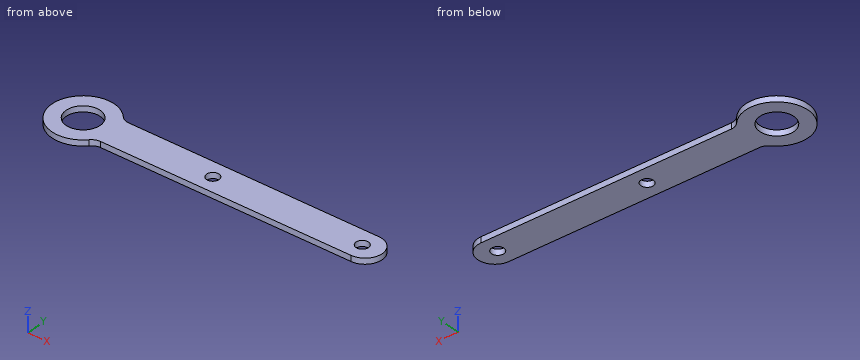
Autodesk Inventor part; units mm, degrees
ref_plane "YZ Plane" through (0, 0, 0) normal (1, 0, 0) x (0, 1, 0)
ref_plane "XZ Plane" through (0, 0, 0) normal (0, 1, 0) x (-1, 0, 0)
ref_plane "XY Plane" through (0, 0, 0) normal (0, 0, 1) x (1, 0, 0)
sketch "Skizze1" plane through (0, 0, 0) normal (0, 0, 1) x (1, 0, 0)
  line L0 (0, 0) -> (38.7995, 0) construction
  arc A0 (4.6098, 3) -> (4.6098, -3) centre (0, 0) ccw
  circle A1 centre (0, 0) radius 3
  line L1 (4.6098, 3) -> (4.6098, -3)
  line L2 (4.6098, 3) -> (50, 3)
  line L3 (53, 0) -> (53, 0)
  line L4 (50, -3) -> (4.6098, -3)
  arc A2 (53, 0) -> (50, 3) centre (50, 0) ccw
  arc A3 (50, -3) -> (53, 0) centre (50, 0) ccw
  point P0 (53, 0)
  dimension "d1" = 6
  dimension "d4" = 6
  dimension "d5" = 5.5
  dimension "d6" = 3
  dimension "d7" = 50
extrude "Extrusion1" add sketch "Skizze1" along normal blind 1
fillet "Rundung1" radius 2 2 edges at (4.6098, 3, 0.5) (4.6098, -3, 0.5)
sketch "Skizze3" plane through (0, 0, 0) normal (0, 0, -1) x (-1, 0, 0)
  point P0 (0, 0)
  point P1 (-49.5, 0)
  dimension "d26" = 49.5
hole "Bohrung2" at (49.5, 0, 0) direction (0, 0, 1) diameter 2.2 depth 1
sketch "Skizze2" plane through (0, 0, 1) normal (0, 0, 1) x (1, 0, 0)
  point P0 (0, 0)
  point P1 (23, 0)
  dimension "d18" = 23
hole "Bohrung1" at (23, 0, 1) direction (0, 0, -1) diameter 2.2 depth 1
properties part number "pleuel" material "Edelstahl, 440C"
CAD build for the part. Positions are in the model's coordinates, mm. Coordinates: 2 decimals unless noted, no trailing zeros. Order: outer loops, then holes, each group sorted by start corner. A loop starts at its lowest first (then second) coordinate and runs counter-clockwise, first axis right, second up. Notation, with made-up numbers: (69, 41) - (122, 41) arc R37 cw to (122, 79) - close; hole circle Ø9 at (77, 59). An arc over 180 degrees is marked (long way). Use a Markdown table: item, result. Add a question column.
(1) Saw through at C-C (z = 0.45). Give the cut face in (x, y).
(2) Drill centre lines: line 1 along Y through (x, z) = (49.5, 0.45); line 2 along Y through (x, z) = (0, 0.6); line 3 along X through (y, z) = (-0.75, 0.5). Where is each one in solid material? Low to high. Write a range as [from, to].
(3) Saw through at B-B (y = 0). Give the cut face in (x, z), then the cut area to 3 significant figures.
(4) Saw through at D-D (x = 0). Give the cut face in (y, z), then the cut area to 3 significant figures.
(5) Flat gauge pin, fed straight in: pin 1 (1.8 mm diameter, centred on x = 23, y = 0, fed in from -Z). Where does the tip first touch, or does it go through?
(6) Saw through at A-A (x = 49.5). Give the cut face in (y, z).
Solved:
| question | item | result |
|---|---|---|
| 1 | outline | (4.1, -3.67) arc R2 cw to (5.59, -3) - (50, -3) arc R3 ccw to (50, 3) - (5.59, 3) arc R2 cw to (4.1, 3.67) arc R5.5 ccw (long way) to start; hole circle Ø6 at (0, 0); hole circle Ø2.2 at (23, 0); hole circle Ø2.2 at (49.5, 0) |
| 2 | line 1 | y = [-3, -1.1], [1.1, 3] |
| 2 | line 2 | y = [-5.5, -3], [3, 5.5] |
| 2 | line 3 | x = [-5.45, -2.9], [2.9, 22.2], [23.8, 48.7], [50.3, 52.9] |
| 3 | outline | (-5.5, 0) - (-3, 0) - (-3, 1) - (-5.5, 1) - close; (3, 0) - (21.9, 0) - (21.9, 1) - (3, 1) - close; (24.1, 0) - (48.4, 0) - (48.4, 1) - (24.1, 1) - close; (50.6, 0) - (53, 0) - (53, 1) - (50.6, 1) - close |
| 3 | area | 48.1 mm² |
| 4 | outline | (-5.5, 0) - (-3, 0) - (-3, 1) - (-5.5, 1) - close; (3, 0) - (5.5, 0) - (5.5, 1) - (3, 1) - close |
| 4 | area | 5.00 mm² |
| 5 | pin 1 | passes through |
| 6 | outline | (-3, 0) - (-1.1, 0) - (-1.1, 1) - (-3, 1) - close; (1.1, 0) - (3, 0) - (3, 1) - (1.1, 1) - close |
